CAD build for the part. Positions are in the model's coordinates, mm. Round coordinates to 2 decimals unless told otherwise and drop trailing zeros. Write each loop counter-clockwise with the first axis right and the second up, starting at its lowest first coordinate (ties: lowest second). Pieces come first, ordered by that corner, then holes. Notation, with made-up numbers: (-29, 39) -> (6, 39) arc R29 cw to (6, 78) -> close; hole circle Ø8 at (-27.75, 11). An arc over 180 degrees is marked (long way). Put each result on its own line as item: value. Start each with the question number.
1. Saw through at C-C on x = 8.5. List the corners of the cut face in (y, z).
2. Saw through at B-B on z = 17. List the corners of the cut face in (x, y) (1 decimal).
3. Drill centre lines: line 1 (Y direction, x = 23, z = 20.5); line 2 (X direction, y = -3, z = 5); line 3 (Y direction, x = 7.5, z = 20). Where is each one in solid material? Low to high. Write a range as from..to.
4. Pull direction X, two halves, no side cores. Call faces 1 (the flat face through (47, 17, 0)), 2 (the flat face through (2.15, -9.62, 19.72)), 3 (the flat face through (64.349, 43.442, 14.916)): pulls with the +X half, pulls with the -X half, needs draft (parallel to the pull), parting line crosses it, or undercut.
5. Flat gauge pins, fed straight in: P1, Ø5, axis at x = 19.5, y = 31.5, coming from the -Z side; P2, Ø16, axis at x = 11.05, y = -7.25, coming from the +Z side; P3, Ø12, axis at y = -4, z = 13, coming from the +X side; P4, Ø4, axis at x = 41, z = 33.5, coming from the +Y side. Where does each tip first touch, or does it go through?
6. Saw through at A-A on y = -5. List the corners of the cut face in (x, z).
7. Saw through at D-D on x = 32. State how many separate pieces and enclosed holes the cut face has, and give its area (3 significant figures).
from build123d import *

# Parameters (mm, degrees)
BOSS_EXTRUDE1_DEPTH     = 40
CUT_EXTRUDE1_DEPTH      = 111.69728555
CUT_EXTRUDE1_DEPTH_BACK = 111.69728555
SKETCH3_R               = 5
SWEEP3_PROFILE_R        = 6
SWEEP4_PROFILE_R        = 6


with BuildPart() as part:
    # Sketch1 → Boss-Extrude1 (new body)
    with BuildSketch(Plane.XY):
        with BuildLine():
            Line((0, 0), (4.364992014, -19.517859635))
            ThreePointArc((4.364992014, -19.517859635), (53.125172498, 2.703315983), (88.780401421, 42.703822193))
            Line((88.780401421, 42.703822193), (71.428423344, 52.649115393))
            ThreePointArc((71.428423344, 52.649115393), (41.258614256, 18.802533215), (0, 0))
        make_face()
    extrude(amount=BOSS_EXTRUDE1_DEPTH)

    # Sketch3 → Cut-Extrude1 (cut, two sides: drawn at the far end of the back side and taken through both)
    with BuildSketch(Plane.XY.offset(40).offset(-CUT_EXTRUDE1_DEPTH_BACK)):
        with Locations((11.048099116, -7.247975554)):
            Circle(SKETCH3_R)
    extrude(amount=CUT_EXTRUDE1_DEPTH + CUT_EXTRUDE1_DEPTH_BACK, mode=Mode.SUBTRACT)

    # Sweep3: sweep along a path in Sketch32
    with BuildLine(Plane.XY.offset(15)) as sweep3_path:
        ThreePointArc((65.395294118, 44.437442075), (48.35413652, 57.815528603), (28.200002322, 65.764435832))
    # Sweep3 profile (on start of the path) → Sweep3 (sweep)
    with BuildSketch(Plane(origin=(65.395294118, 44.437442075, 15), x_dir=(0.7246292666888544, 0.6891389017157377, 0), z_dir=(-0.6891389017157377, 0.7246292666888544, 0))):
        Circle(SWEEP3_PROFILE_R)
    sweep(path=sweep3_path.line)

    # Sweep4: sweep along a path in Sketch48
    with BuildLine(Plane.XY.offset(15)) as sweep4_path:
        ThreePointArc((51.136783714, 14.042285968), (38.184106553, 28.895053348), (20.126776716, 36.788682657))
    # Sweep4 profile (on start of the path) → Sweep4 (sweep)
    with BuildSketch(Plane(origin=(51.136783714, 14.042285968, 15), x_dir=(0.879297732143527, 0.47627250418982864, 0), z_dir=(-0.47627250418982864, 0.879297732143527, 0))):
        Circle(SWEEP4_PROFILE_R)
    sweep(path=sweep4_path.line)


solid = part.part
Return value:
1. outline: (-18.52, 0) -> (-11.55, 0) -> (-11.55, 40) -> (-18.52, 40) -> close; (-2.95, 0) -> (2.26, 0) -> (2.26, 40) -> (-2.95, 40) -> close
2. outline: (0, 0) -> (4.4, -19.5) arc R130 ccw to (88.8, 42.7) -> (71.4, 52.6) arc R110 cw to (69.1, 48.8) arc R80.7 ccw to (29.5, 71.3) -> (26.9, 60.3) arc R69.3 cw to (61.3, 40.5) -> (67.7, 46.7) arc R110 cw to (49.8, 25.8) arc R50.7 ccw to (21.2, 42.3) -> (19.1, 31.2) arc R39.3 cw to (41.1, 18.7) arc R110 cw to start; hole circle Ø10 at (11, -7.2)
3. line 1: y = -13.86..7.9, 33.65..38.61
3. line 2: x = 0.67..8.41, 13.69..44.72
3. line 3: y = -18.78..-10.77, -3.73..1.96
4. face 1: needs draft
4. face 2: pulls with the -X half
4. face 3: undercut
5. P1: stops at z = 9.7
5. P2: stops at z = 40
5. P3: stops at x = 52.16
5. P4: stops at y = 20.11
6. outline: (1.12, 0) -> (6.58, 0) -> (6.58, 40) -> (1.12, 40) -> close; (15.51, 0) -> (41.4, 0) -> (41.4, 40) -> (15.51, 40) -> close
7. separate pieces: 3
7. enclosed holes: 0
7. area: 1,150 mm^2
